CAD build for the part. Positions are in the model's coordinates, mm. Round coordinates to 2 decimals unless told otherwise and drop trailing zeros. Write each loop counter-clockwise with the first axis right and the second up, starting at its lowest first coordinate (ties: lowest second). Pieces come first, ordered by that corner, then holes. Notation, with made-up numbers: (74, 50) - (109, 50) arc R19 ccw to (109, 60) - close; hole circle Ø9 at (-23.5, 1.5). An arc over 180 degrees is marked (long way). Put each result on its own line as item: value. Start each with the question number.
Item 1: Cut at B-B (z = -32). Give the cut face in (x, y), and give its area (3 significant figures).
Item 2: Cut at A-A (x = 0). Give the cut face in (y, z).
Item 3: Cut at D-D (y = 1.7). Count the separate pieces of the cut face and the enclosed holes in it, and give its area (3 significant figures).
Item 4: Pin check, flat tip, straight feed: pin 1 Ø2.5 at (x, z) = (11.67, 11.67) entering from +Y. Stop position of the tip, or through.
Item 5: Cut at C-C (z = -8.5). Give the cut face in (x, y).
Item 6: Mould opens along Z. For faces 1 (the flat face through (0, 1, -39.5)), 2 (the flat face through (20.5, 1, -17)), 3 (the cylindrical face through (-12.28, 0.986, 13.145)) say: released by +Z, released by -Z, zero draft, split by the parting line, or undercut.
Item 7: Drill centre lines: line 1 (X direction, y = 1.25, z = -32.5); line 2 (X direction, y = 1.15, z = 11); line 3 (X direction, y = 1, z = -8.5). Where is each one in solid material? Low to high. Write a range as from..to.
```python
from build123d import *

# Parameters (mm, degrees)
SKETCH_1_R      = 1.6
SKETCH_1_R_2    = 20.5
SKETCH_1_R_3    = 12.5
SKETCH_1_R_4    = 3.6
EXTRUDE_1_DEPTH = 2
FILLET_1_R      = 5


with BuildPart() as part:
    # 草图1 → 凸台-拉伸1 (new body)
    # profile 1 of 3: a face of its own
    with BuildSketch(Plane(origin=(0, 0, 0), x_dir=(1, 0, 0), z_dir=(0, 1, 0))):
        with BuildLine():
            Line((-20.5, 39.5), (-20.5, 0))
            ThreePointArc((-20.5, 0), (0, 20.5), (20.5, 0))
            Line((20.5, 0), (20.5, 39.5))
            Line((20.5, 39.5), (-20.5, 39.5))
        make_face()
        with Locations(Location((-10, 32, 0), (0, 0, 270))):
            Circle(SKETCH_1_R, mode=Mode.SUBTRACT)
        with Locations(Location((10, 32, 0), (0, 0, 270))):
            Circle(SKETCH_1_R, mode=Mode.SUBTRACT)
    # profile 2 of 3: a face of its own
    with BuildSketch(Plane(origin=(0, 0, 0), x_dir=(1, 0, 0), z_dir=(0, 1, 0))):
        Circle(SKETCH_1_R_2)
        with Locations(Location((11.66726189, -11.66726189, 0), (0, 0, 270))):
            Circle(SKETCH_1_R, mode=Mode.SUBTRACT)
        with Locations(Location((11.66726189, 11.66726189, 0), (0, 0, 270))):
            Circle(SKETCH_1_R, mode=Mode.SUBTRACT)
        with Locations(Location((-11.66726189, 11.66726189, 0), (0, 0, 270))):
            Circle(SKETCH_1_R, mode=Mode.SUBTRACT)
        with Locations(Location((-11.66726189, -11.66726189, 0), (0, 0, 270))):
            Circle(SKETCH_1_R, mode=Mode.SUBTRACT)
        Circle(SKETCH_1_R_3, mode=Mode.SUBTRACT)
    # profile 3 of 3: a face of its own
    with BuildSketch(Plane(origin=(0, 0, 0), x_dir=(1, 0, 0), z_dir=(0, 1, 0))):
        Circle(SKETCH_1_R_3)
        with Locations(Location((0, -8.5, 0), (0, 0, 270))):
            Circle(SKETCH_1_R, mode=Mode.SUBTRACT)
        with Locations(Location((0, 8.5, 0), (0, 0, 270))):
            Circle(SKETCH_1_R, mode=Mode.SUBTRACT)
        with Locations(Location((0, 0, 0), (0, 0, 270))):
            Circle(SKETCH_1_R_4, mode=Mode.SUBTRACT)
    extrude(amount=EXTRUDE_1_DEPTH)

    # 圆角1
    fillet_1_edges = [part.edges().sort_by_distance(p)[0] for p in [
        (-20.5, 1, -39.5),
        (20.5, 1, -39.5),
    ]]
    fillet(fillet_1_edges, radius=FILLET_1_R)


solid = part.part
```
Output values:
1. outline: (-20.5, 0) - (-11.6, 0) - (-11.6, 2) - (-20.5, 2) - close; (-8.4, 0) - (8.4, 0) - (8.4, 2) - (-8.4, 2) - close; (11.6, 0) - (20.5, 0) - (20.5, 2) - (11.6, 2) - close
1. area: 69.2 mm2
2. outline: (0, -39.5) - (2, -39.5) - (2, -10.1) - (0, -10.1) - close; (0, -6.9) - (2, -6.9) - (2, -3.6) - (0, -3.6) - close; (0, 3.6) - (2, 3.6) - (2, 6.9) - (0, 6.9) - close; (0, 10.1) - (2, 10.1) - (2, 20.5) - (0, 20.5) - close
3. separate pieces: 1
3. enclosed holes: 9
3. area: 2,160 mm2
4. pin 1: through
5. outline: (-20.5, 0) - (-1.6, 0) - (-1.6, 2) - (-20.5, 2) - close; (1.6, 0) - (20.5, 0) - (20.5, 2) - (1.6, 2) - close
6. face 1: released by -Z
6. face 2: zero draft
6. face 3: undercut
7. line 1: -20.5..-11.52, -8.48..8.48, 11.52..20.5
7. line 2: -17.3..-13.12, -10.21..10.21, 13.12..17.3
7. line 3: -20.5..-1.6, 1.6..20.5
